Part print with two shaded views. Sizes in mm from the minimum x, y, z corner. A direction names the side the tool comes from. Give positions to 0.01 mm unless a question says otherwise; leave off trailing zeros. Write each loop counter-clockwise with the first axis right and the second up, starting at its lowest first coordinate (ties: lowest second). Pieces come first, ordered by that corner, then holes.
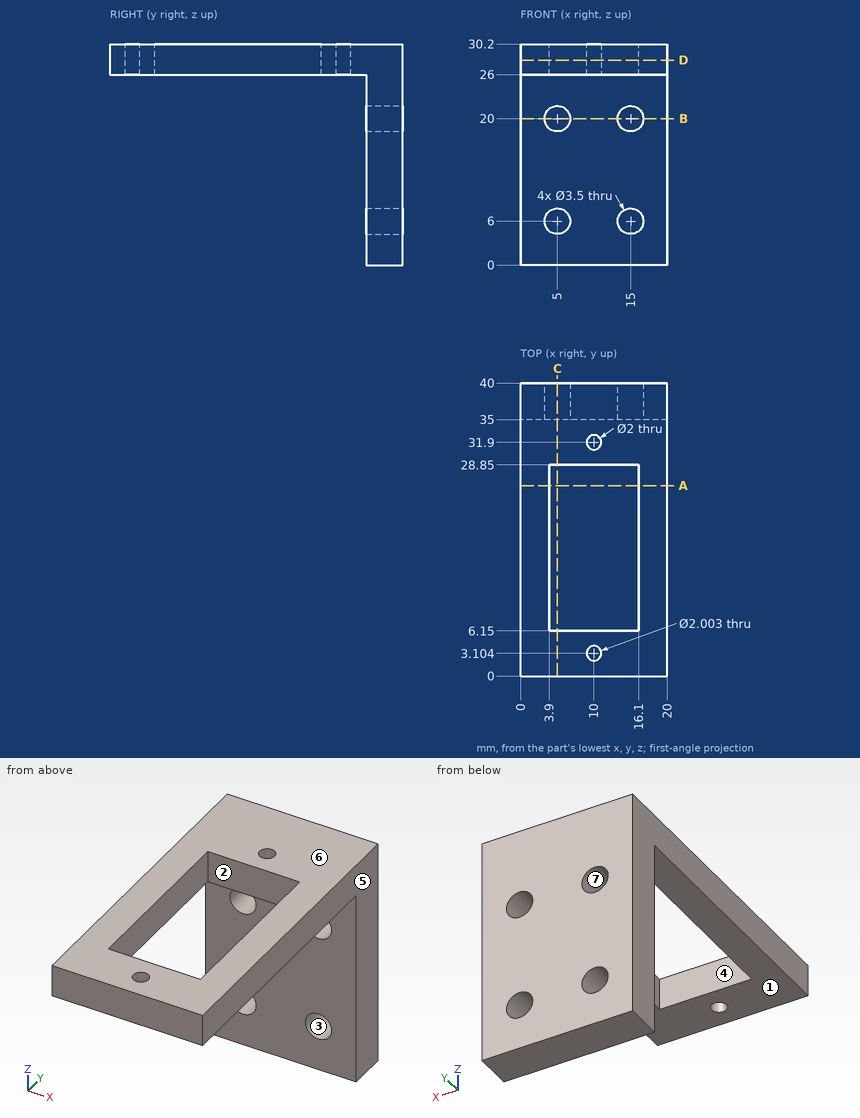
1) Saw through at C-C (x = 5). Write the cut outline in (y, z), and give its area (3 significant figures).
Check result:
outline: (0, 26) - (6.15, 26) - (6.15, 30.2) - (0, 30.2) - close; (28.85, 26) - (35, 26) - (35, 21.75) - (40, 21.75) - (40, 30.2) - (28.85, 30.2) - close; (35, 0) - (40, 0) - (40, 4.25) - (35, 4.25) - close; (35, 7.75) - (40, 7.75) - (40, 18.25) - (35, 18.25) - close
area: 168 mm2
2) Saw through at B-B (z = 20). Write the cut outline in (x, y), and give its area (3 significant figures).
Check result:
outline: (0, 35) - (3.25, 35) - (3.25, 40) - (0, 40) - close; (6.75, 35) - (13.25, 35) - (13.25, 40) - (6.75, 40) - close; (16.75, 35) - (20, 35) - (20, 40) - (16.75, 40) - close
area: 65.0 mm2
3) 3-axis set-ups, long thin cutter, end or side, ignore diameter. For the marked faces 1, 2 and 3: which of +Z, -Z, +X, -X, +Y, -Y reach the whole face in a straight line?
Check result:
face 1: -Z, +X, -X, -Y
face 2: +Z, -Z
face 3: +Y, -Y
4) Drill centre lines: L1, parallel to Z at x = 5, y = 38.5; L2, parallel to X at y = 36, z = 6; L3, parallel to Z at x = 4, y = 6. Where is each one in solid material? Low to high.
Check result:
L1: z = 0 to 4.25, 7.75 to 18.25, 21.75 to 30.2
L2: x = 0 to 3.25, 6.75 to 13.25, 16.75 to 20
L3: z = 26 to 30.2
5) Saw through at A-A (y = 26). Write the cut outline in (x, z).
Check result:
outline: (0, 26) - (3.9, 26) - (3.9, 30.2) - (0, 30.2) - close; (16.1, 26) - (20, 26) - (20, 30.2) - (16.1, 30.2) - close
6) Saw through at D-D (z = 28). Write the cut outline in (x, y).
Check result:
outline: (0, 0) - (20, 0) - (20, 40) - (0, 40) - close; hole (3.9, 6.15) - (16.1, 6.15) - (16.1, 28.85) - (3.9, 28.85) - close; hole circle Ø2 at (10, 3.1); hole circle Ø2 at (10, 31.9)
7) Flat gauge pins, fed straight in: P1, Ø6, axis at x = 9, y = 9.5, coming from the +Z side; P2, Ø2, axis at x = 15.5, y = 10.5, coming from the -Z side; P3, Ø5.5, axis at x = 5, z = 20, coming from the -Y side. Where does each tip first touch, or does it go through?
Check result:
P1: passes through
P2: stops at z = 26
P3: stops at y = 35
8) Mould opens along X. For the marked faces 4, 5, 6 and 7 say: +X half, -X half, draft (parallel to the pull), parting line (faces both ways), or undercut.
Check result:
face 4: undercut
face 5: +X half
face 6: draft
face 7: undercut
